```python
from build123d import *

# Parameters (mm, degrees)
SKETCH1_R           = 31.031300013
SKETCH1_R_2         = 3.067047094
EXTRUDE3_DEPTH      = 5
EXTRUDE3_DEPTH_BACK = 5
SKETCH1_6_R         = 62.603843631
SKETCH1_6_R_2       = 31.031300013
EXTRUDE4_DEPTH      = 30
EXTRUDE4_DEPTH_BACK = 30


with BuildPart() as part:
    # Sketch1 → Extrude3 (new body, two sides)
    with BuildSketch(Plane.XY) as extrude3_sk:
        Circle(SKETCH1_R)
        Circle(SKETCH1_R_2, mode=Mode.SUBTRACT)
    extrude(amount=EXTRUDE3_DEPTH)
    extrude(extrude3_sk.sketch, amount=-EXTRUDE3_DEPTH_BACK)

    # Sketch1_6 → Extrude4 (add, two sides)
    with BuildSketch(Plane.XY) as extrude4_sk:
        Circle(SKETCH1_6_R)
        Circle(SKETCH1_6_R_2, mode=Mode.SUBTRACT)
    extrude(amount=EXTRUDE4_DEPTH)
    extrude(extrude4_sk.sketch, amount=-EXTRUDE4_DEPTH_BACK)


solid = part.part
```
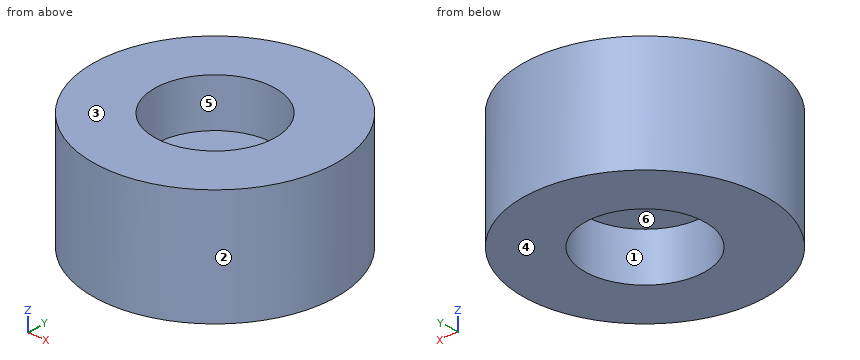
Model file for the job. Use its own axes, mm. Face numbers are marked on the shaded views. A direction names the side the tool comes from. Coordinates: 2 decimals unless noted, no trailing zeros. Loops run counter-clockwise (first coordinate to the right, second up) from the corner with the lowest first, then second, coordinate; pieces in that order, holes last. Notation, with made-up numbers: (12, 25) -> (32, 25) arc R27 cw to (32, 57) -> close; hole circle Ø6 at (60, 52). An arc over 180 degrees is marked (long way). Answer as a JSON object with one key per item and string values.
Q1. Flat gauge pins, fed straight in: P1, Ø8, axis at x = 0, y = 0, coming from the +Z side; P2, Ø1, axis at y = 25.5, z = -5, coming from the +X side; P3, Ø2, axis at y = -21.5, z = -19, coming from the -X side. Where does each tip first touch, or does it go through?
Report:
{"P1": "stops at z = 5", "P2": "stops at x = 57.4", "P3": "stops at x = -59.15"}
Q2. Cut at A-A (y = 0). List the corners of the cut face in (x, z).
Report:
{"outline": "(-62.6, -30) -> (-31.03, -30) -> (-31.03, -5) -> (-3.07, -5) -> (-3.07, 5) -> (-31.03, 5) -> (-31.03, 30) -> (-62.6, 30) -> close; (3.07, -5) -> (31.03, -5) -> (31.03, -30) -> (62.6, -30) -> (62.6, 30) -> (31.03, 30) -> (31.03, 5) -> (3.07, 5) -> close"}
Q3. Pull direction Y, two halves, no side cores. Call the marked faces 1, 2 and 3: released by +Y, released by -Y, zero draft, split by the parting line, or undercut.
Report:
{"face 1": "undercut", "face 2": "split by the parting line", "face 3": "zero draft"}
Q4. Cut at C-C (z = -13). List the corners of the cut face in (x, y).
Report:
{"outline": "circle Ø125.21 at (0, 0); hole circle Ø62.06 at (0, 0)"}
Q5. Cut at D-D (y = 13.5). List the corners of the cut face in (x, z).
Report:
{"outline": "(-61.13, -30) -> (-27.94, -30) -> (-27.94, -5) -> (27.94, -5) -> (27.94, -30) -> (61.13, -30) -> (61.13, 30) -> (27.94, 30) -> (27.94, 5) -> (-27.94, 5) -> (-27.94, 30) -> (-61.13, 30) -> close"}
Q6. 3-axis set-ups, long thin cutter, end or side, ignore diameter. For the marked faces 4, 5 and 6: which of +Z, -Z, +X, -X, +Y, -Y reach the whole face in a straight line?
Report:
{"face 4": "-Z, +X, -X, +Y, -Y", "face 5": "+Z", "face 6": "-Z"}
Q7. Probe probe 1 along Y at (x, z) = (0, 13.25); probe 2 along Y at (x, z) = (0, -1.25); probe 3 along Z at (x, y) = (-18, 11). List the from-to ranges inside material, lowest first.
Report:
{"probe 1": "y = -62.6 to -31.03, 31.03 to 62.6", "probe 2": "y = -62.6 to -3.07, 3.07 to 62.6", "probe 3": "z = -5 to 5"}
